```python
from build123d import *

# Parameters (mm, degrees)
SKETCH1_W           = 33
SKETCH1_H           = 23
BOSS_EXTRUDE1_DEPTH = 10
SKETCH2_W           = 10
SKETCH2_H           = 23
BOSS_EXTRUDE2_DEPTH = 23
SKETCH3_R           = 2
CUT_EXTRUDE1_DEPTH  = 33
SKETCH4_R           = 2
CUT_EXTRUDE2_DEPTH  = 33
BOSS_EXTRUDE3_DEPTH = 23
SKETCH6_R           = 3.5
CUT_EXTRUDE3_DEPTH  = 33
SKETCH7_R           = 3.5
CUT_EXTRUDE4_DEPTH  = 33
SKETCH8_W           = 33
SKETCH8_H           = 11.5
CUT_EXTRUDE5_DEPTH  = 53


with BuildPart() as part:
    # Sketch1 → Boss-Extrude1 (new body)
    with BuildSketch(Plane.XY):
        with Locations((-15.439393939, -2.291666667)):
            Rectangle(SKETCH1_W, SKETCH1_H)
    extrude(amount=BOSS_EXTRUDE1_DEPTH)

    # Sketch2 → Boss-Extrude2 (add)
    with BuildSketch(Plane.XY.offset(10)):
        with Locations((-3.939393939, -2.291666667)):
            Rectangle(SKETCH2_W, SKETCH2_H)
    extrude(amount=BOSS_EXTRUDE2_DEPTH)

    # Sketch3 → Cut-Extrude1 (cut)
    with BuildSketch(Plane.XY.offset(10)):
        with Locations((-24.939393939, 3.208333333)):
            Circle(SKETCH3_R)
        with Locations((-24.939393939, -7.791666667)):
            Circle(SKETCH3_R)
    extrude(amount=-CUT_EXTRUDE1_DEPTH, mode=Mode.SUBTRACT)

    # Sketch4 → Cut-Extrude2 (cut)
    with BuildSketch(Plane.ZY.offset(8.939393939)):
        with Locations(Location((26, 3.208333333, 0), (0, 0, 270))):
            Circle(SKETCH4_R)
        with Locations(Location((26, -7.791666667, 0), (0, 0, 270))):
            Circle(SKETCH4_R)
    extrude(amount=-CUT_EXTRUDE2_DEPTH, mode=Mode.SUBTRACT)

    # Sketch5 → Boss-Extrude3 (add)
    with BuildSketch(Plane(origin=(0, -13.791666667, 0), x_dir=(-1, 0, 0), z_dir=(0, -1, 0))):
        Polygon((8.939393939, -10), (8.939393939, -33), (31.939393939, -10), align=None)
    extrude(amount=-BOSS_EXTRUDE3_DEPTH)

    # Sketch6 → Cut-Extrude3 (cut)
    with BuildSketch(Plane(origin=(-8.939393939, 0, 0), x_dir=(0, 0, -1), z_dir=(1, 0, 0))):
        with Locations((-26, -7.791666667)):
            Circle(SKETCH6_R)
        with Locations((-26, 3.208333333)):
            Circle(SKETCH6_R)
    extrude(amount=-CUT_EXTRUDE3_DEPTH, mode=Mode.SUBTRACT)

    # Sketch7 → Cut-Extrude4 (cut)
    with BuildSketch(Plane(origin=(0, 0, 10), x_dir=(-1, 0, 0), z_dir=(0, 0, -1))):
        with Locations((24.939393939, -7.791666667)):
            Circle(SKETCH7_R)
        with Locations((24.939393939, 3.208333333)):
            Circle(SKETCH7_R)
    extrude(amount=-CUT_EXTRUDE4_DEPTH, mode=Mode.SUBTRACT)

    # Sketch8 → Cut-Extrude5 (cut)
    with BuildSketch(Plane.ZY.offset(31.939393939)):
        with Locations((16.5, 3.458333333)):
            Rectangle(SKETCH8_W, SKETCH8_H)
    extrude(amount=-CUT_EXTRUDE5_DEPTH, mode=Mode.SUBTRACT)


solid = part.part
```
Part model, mm, in its own coordinate system. A direction names the side the tool comes from. Round coordinates to 2 decimals unless told otherwise and drop trailing zeros. Loops run counter-clockwise (first coordinate to the right, second up) from the corner with the lowest first, then second, coordinate; pieces in that order, holes last. Notation, with made-up numbers: (-21.75, -31.75) -> (30.25, -31.75) arc R6 ccw to (30.25, -25.75) -> close; hole circle Ø11 at (-3.5, 38.5). An arc over 180 degrees is marked (long way). Use a Markdown table: item, result.
1) Cut at B-B, the plane y = -3.5. List the corners of the cut face in (x, z), and give its area (4 significant figures).
The answers:
| item | result |
|---|---|
| outline | (-31.94, 0) -> (1.06, 0) -> (1.06, 33) -> (-8.94, 33) -> (-31.94, 10) -> close |
| area | 824.5 mm2 |
2) Tool access for faces 4 (the cylindrical face through (-21.443, -7.638, 14.065)), 5 (the flat face through (-8.939, -9, 24)), 6 (the cylindrical face through (-4.009, -7.358, 24.048)): list every direction of +Z, -Z, +X, -X, +Y, -Y with a clear straight run to the whole face (end or side of a thin tool).
The answers:
| item | result |
|---|---|
| face 4 | +Z |
| face 5 | -X |
| face 6 | +X, -X |
3) Cut at A-A, the plane z = 26. List the corners of the cut face in (x, y), and give its area (4 significant figures).
The answers:
| item | result |
|---|---|
| outline | (-15.94, -13.79) -> (1.06, -13.79) -> (1.06, -9.79) -> (-8.94, -9.79) -> (-8.94, -11.29) -> (-15.94, -11.29) -> close; (-15.94, -4.29) -> (-8.94, -4.29) -> (-8.94, -5.79) -> (1.06, -5.79) -> (1.06, -2.29) -> (-15.94, -2.29) -> close |
| area | 106.5 mm2 |
4) Probe line 1 (X direction, y = -5, z = 13); line 2 (X direction, y = -11, z = 27); line 3 (X direction, y = -8.25, z = 13). List the from-to ranges inside material, lowest first. Write a range as [from, to].
The answers:
| item | result |
|---|---|
| line 1 | x = [-28.94, -27.05], [-22.83, 1.06] |
| line 2 | x = [-8.94, 1.06] |
| line 3 | x = [-28.94, -28.41], [-21.47, 1.06] |
5) Drop flat-ended pins along their axis: pin 1 Ø3.5 at (x, y) = (-23.5, -7.5) entering from +Z; pin 2 Ø2 at (y, z) = (-9, 25) entering from -X; pin 3 Ø5 at (x, z) = (-16.5, 26.5) entering from +Y; pin 4 Ø1.5 at (x, y) = (-10.5, -8.5) entering from +Z. Give the stop position or say it passes through.
The answers:
| item | result |
|---|---|
| pin 1 | stops at z = 10 |
| pin 2 | stops at x = -8.94 |
| pin 3 | stops at y = -2.29 |
| pin 4 | stops at z = 32.19 |
6) Pull direction X, two halves, no side cores. Call faces 1 (the cylindrical face through (-23.03, -7.19, 5.07)), 2 (the flat face through (-20.28, -8.12, 21.66)), 3 (the flat face through (-12, -2.292, 13)): pulls with the +X half, pulls with the -X half, needs draft (parallel to the pull), parting line crosses it, or undercut.
The answers:
| item | result |
|---|---|
| face 1 | undercut |
| face 2 | pulls with the -X half |
| face 3 | needs draft |
7) Cut at C-C, the plane x = -28. List the corners of the cut face in (y, z).
The answers:
| item | result |
|---|---|
| outline | (-13.79, 0) -> (-2.29, 0) -> (-2.29, 13.94) -> (-6.09, 13.94) -> (-6.09, 10) -> (-9.49, 10) -> (-9.49, 13.94) -> (-13.79, 13.94) -> close |
8) Cut at D-D, the plane z = 13. List the corners of the cut face in (x, y).
The answers:
| item | result |
|---|---|
| outline | (-28.94, -13.79) -> (1.06, -13.79) -> (1.06, -2.29) -> (-28.94, -2.29) -> close; hole circle Ø7 at (-24.94, -7.79) |
